For this review, take the finished solid that the model builds, in its own axes (mm). Give positions to 0.01 mm unless a question says otherwise; leave off trailing zeros. Loops run counter-clockwise (first coordinate to the right, second up) from the corner with the lowest first, then second, coordinate; pieces in that order, holes last. Notation, with made-up numbers: (57, 34.25) - (80, 34.25) arc R20 ccw to (80, 60.25) - close; hole circle Ø7 at (34, 14.5). An arc over 180 degrees is marked (long way). Answer as CSV lines item,"result".
from build123d import *

# Parameters (mm, degrees)
SKETCH1_W           = 300
SKETCH1_H           = 120
SKETCH1_R           = 4
SKETCH1_R_2         = 1.5
SKETCH1_W_2         = 14
SKETCH1_H_2         = 14
BOSS_EXTRUDE1_DEPTH = 2


with BuildPart() as part:
    # Sketch1 → Boss-Extrude1 (new body)
    with BuildSketch(Plane(origin=(0, 0, 0), x_dir=(1, 0, 0), z_dir=(0, 1, 0))):
        Rectangle(SKETCH1_W, SKETCH1_H)
        with Locations(Location((-95, 0, 0), (0, 0, 270))):
            Circle(SKETCH1_R, mode=Mode.SUBTRACT)
        with Locations(Location((-145, 55, 0), (0, 0, 270))):
            Circle(SKETCH1_R_2, mode=Mode.SUBTRACT)
        with Locations(Location((145, 55, 0), (0, 0, 90))):
            Circle(SKETCH1_R_2, mode=Mode.SUBTRACT)
        with Locations(Location((-145, -55, 0), (0, 0, 90))):
            Circle(SKETCH1_R_2, mode=Mode.SUBTRACT)
        with Locations(Location((145, -55, 0), (0, 0, 270))):
            Circle(SKETCH1_R_2, mode=Mode.SUBTRACT)
        with Locations(Location((5, 55, 0), (0, 0, 270))):
            Circle(SKETCH1_R_2, mode=Mode.SUBTRACT)
        with Locations(Location((5, -55, 0), (0, 0, 90))):
            Circle(SKETCH1_R_2, mode=Mode.SUBTRACT)
        with Locations((24.5, -40)):
            Rectangle(SKETCH1_W_2, SKETCH1_H_2, mode=Mode.SUBTRACT)
        with Locations((40, 3)):
            Rectangle(SKETCH1_W_2, SKETCH1_H_2, mode=Mode.SUBTRACT)
        with Locations((71, 3)):
            Rectangle(SKETCH1_W_2, SKETCH1_H_2, mode=Mode.SUBTRACT)
        with Locations((102, 3)):
            Rectangle(SKETCH1_W_2, SKETCH1_H_2, mode=Mode.SUBTRACT)
        with Locations((55.5, -40)):
            Rectangle(SKETCH1_W_2, SKETCH1_H_2, mode=Mode.SUBTRACT)
        with Locations((86.5, -40)):
            Rectangle(SKETCH1_W_2, SKETCH1_H_2, mode=Mode.SUBTRACT)
        with Locations((117.5, -40)):
            Rectangle(SKETCH1_W_2, SKETCH1_H_2, mode=Mode.SUBTRACT)
        with Locations((40, 47)):
            Rectangle(SKETCH1_W_2, SKETCH1_H_2, mode=Mode.SUBTRACT)
        with Locations((71, 47)):
            Rectangle(SKETCH1_W_2, SKETCH1_H_2, mode=Mode.SUBTRACT)
        with Locations((102, 47)):
            Rectangle(SKETCH1_W_2, SKETCH1_H_2, mode=Mode.SUBTRACT)
    extrude(amount=BOSS_EXTRUDE1_DEPTH)


solid = part.part
1) Wall thickness on line 1 (Z direction, x = 39.5, y = 0.4); line 2 (X direction, y = 1.2, z = 0); line 3 (X direction, y = 0.9, z = 55): over which ranges is each line inside the solid? List them lowest first. Write a range as from..to.
From the geometry:
line 1,"z = -60..-54, -40..-10, 4..60"
line 2,"x = -150..-99, -91..33, 47..64, 78..95, 109..150"
line 3,"x = -150..-146.5, -143.5..3.5, 6.5..143.5, 146.5..150"
2) Insertion check: P1, Ø3, axis at x = 7.5, z = 9, coming from the -Y side. The pin has a flat end and moves straight along its axis. Give the tip position at first contact, or say it passes through.
From the geometry:
P1,"stops at y = 0"
3) Draft analysis for pull direction Z (two halves, no side actions). For faces 1 (the flat face through (-2, 2, -1)), 2 (the cylindrical face through (-98.905, 0.986, -0.867)), state which applies: pulls with the +Z half, pulls with the -Z half, needs draft (parallel to the pull), parting line crosses it, or undercut.
From the geometry:
face 1,"needs draft"
face 2,"undercut"
4) Consider section A-A on z = 0. Write out the cut boundary in (x, y).
From the geometry:
outline,"(-150, 0) - (-99, 0) - (-99, 2) - (-150, 2) - close; (-91, 0) - (33, 0) - (33, 2) - (-91, 2) - close; (47, 0) - (64, 0) - (64, 2) - (47, 2) - close; (78, 0) - (95, 0) - (95, 2) - (78, 2) - close; (109, 0) - (150, 0) - (150, 2) - (109, 2) - close"
5) Consider section C-C on y = 1.3. Count the separate pieces of the cut face and the enclosed holes in it, and give its area (3 significant figures).
From the geometry:
separate pieces,"1"
enclosed holes,"17"
area,"33,900 mm^2"
6) Consider section B-B on x = -95. Write out the cut boundary in (y, z).
From the geometry:
outline,"(0, -60) - (2, -60) - (2, -4) - (0, -4) - close; (0, 4) - (2, 4) - (2, 60) - (0, 60) - close"
